Read the model definition and answer for the solid it produces. Units are mm, in the model's axes. Face numbers are marked on the shaded views. A direction names the side the tool comes from. Coordinates: 2 decimals unless noted, no trailing zeros. Write each loop counter-clockwise with the first axis right and the second up, starting at its lowest first coordinate (ties: lowest second). Pieces come first, ordered by that corner, then holes.
(1) Determine the mould class of the marked faces 3, 4, 5 and 6 for opening direction Y: pulls with the +Y half, pulls with the -Y half, needs draft (parallel to the pull), parting line crosses it, or undercut.
(2) Which of the six approach directions +Z, -Z, +X, -X, +Y, -Y give full straight-line access (tool end or side, diameter ignored) to the marked faces 1 and 2?
(3) The part is cut by section D-D, the plane z = -21. Determine the outline of the cut face in (x, y), and give its area (3 significant figures).
(4) Straight lines are drawn through the part: line 1 along Y through (x, z) = (0, -4.25); line 2 along Y through (x, z) = (2, -4.75); line 3 along Z through (x, y) = (20.5, -26). For each, find the intervals that lie inside material, in ascending order.
(5) Given pin 1 (1 mm diameter, centred on x = 6, y = 14.5, fed in from +Z); pin 2 (4.5 mm diameter, centred on x = 17.5, y = -17.5, fed in from +Z); pin 3 (4 mm diameter, centred on y = 30, z = -8, fed in from +X), each flat-ended and moving along its own axis, determine where each tip first touches the part or whether it passes through.
(6) The part is cut by section C-C, the plane z = -7.25. State how many separate pieces and enclosed holes the cut face has, and give its area (3 significant figures).
(7) The part is cut by section A-A, the plane x = 0. Determine the outline of the cut face in (y, z).
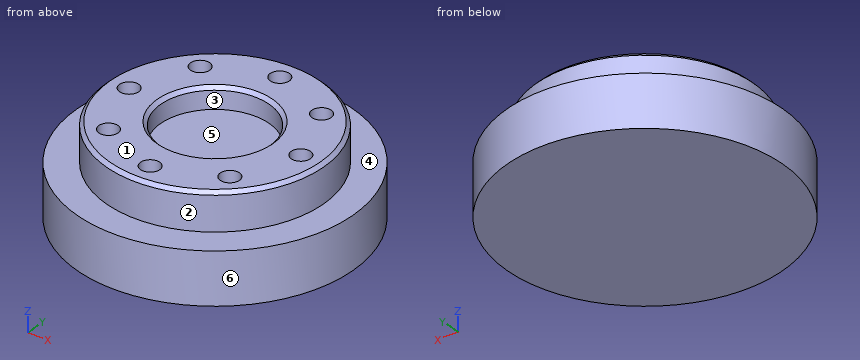
```python
from build123d import *

# Parameters (mm, degrees)
SKETCH1_R           = 31.5
BOSS_EXTRUDE1_DEPTH = 11
SKETCH2_R           = 2.8
CUT_EXTRUDE5_DEPTH  = 9
SKETCH4_R           = 15.75
CUT_EXTRUDE6_DEPTH  = 6.2
CHAMFER1_SIZE       = 1
CHAMFER2_SIZE       = 1
SKETCH5_R           = 40
BOSS_EXTRUDE3_DEPTH = 15


with BuildPart() as part:
    # Sketch1 → Boss-Extrude1 (new body)
    with BuildSketch(Plane.XY):
        Circle(SKETCH1_R)
    extrude(amount=-BOSS_EXTRUDE1_DEPTH)

    # Sketch2 → Cut-Extrude5 (cut)
    with BuildSketch(Plane.XY):
        with Locations((0, 25)):
            Circle(SKETCH2_R)
        with Locations((17.67766953, 17.67766953)):
            Circle(SKETCH2_R)
        with Locations((25, 0)):
            Circle(SKETCH2_R)
        with Locations((17.67766953, -17.67766953)):
            Circle(SKETCH2_R)
        with Locations((0, -25)):
            Circle(SKETCH2_R)
        with Locations((-17.67766953, -17.67766953)):
            Circle(SKETCH2_R)
        with Locations((-25, 0)):
            Circle(SKETCH2_R)
        with Locations((-17.67766953, 17.67766953)):
            Circle(SKETCH2_R)
    extrude(amount=-CUT_EXTRUDE5_DEPTH, mode=Mode.SUBTRACT)

    # Sketch4 → Cut-Extrude6 (cut)
    with BuildSketch(Plane.XY):
        Circle(SKETCH4_R)
    extrude(amount=-CUT_EXTRUDE6_DEPTH, mode=Mode.SUBTRACT)

    # Chamfer1
    chamfer1_edges = [part.edges().sort_by_distance(p)[0] for p in [
        (-31.5, 0, 0),
    ]]
    chamfer(chamfer1_edges, length=CHAMFER1_SIZE)

    # Chamfer2
    chamfer2_edges = [part.edges().sort_by_distance(p)[0] for p in [
        (-15.75, 0, 0),
    ]]
    chamfer(chamfer2_edges, length=CHAMFER2_SIZE)

    # Sketch5 → Boss-Extrude3 (add)
    with BuildSketch(Plane(origin=(0, 0, -11), x_dir=(-1, 0, 0), z_dir=(0, 0, -1))):
        Circle(SKETCH5_R)
    extrude(amount=BOSS_EXTRUDE3_DEPTH)


solid = part.part
```
Computed:
1. face 3: undercut
1. face 4: needs draft
1. face 5: undercut
1. face 6: parting line crosses it
2. face 1: +Z, +X, -X, +Y, -Y
2. face 2: +Z
3. outline: circle Ø80 at (0, 0)
3. area: 5,030 mm2
4. line 1: y = -31.5 to -27.8, -22.2 to -15.75, 15.75 to 22.2, 27.8 to 31.5
4. line 2: y = -31.44 to -26.96, -23.04 to -15.62, 15.62 to 23.04, 26.96 to 31.44
4. line 3: z = -26 to -11
5. pin 1: stops at z = -0.56
5. pin 2: stops at z = -9
5. pin 3: stops at x = 14.43
6. separate pieces: 1
6. enclosed holes: 8
6. area: 2,920 mm2
7. outline: (-40, -26) - (40, -26) - (40, -11) - (31.5, -11) - (31.5, -1) - (30.5, 0) - (27.8, 0) - (27.8, -9) - (22.2, -9) - (22.2, 0) - (16.75, 0) - (15.75, -1) - (15.75, -6.2) - (-15.75, -6.2) - (-15.75, -1) - (-16.75, 0) - (-22.2, 0) - (-22.2, -9) - (-27.8, -9) - (-27.8, 0) - (-30.5, 0) - (-31.5, -1) - (-31.5, -11) - (-40, -11) - close
